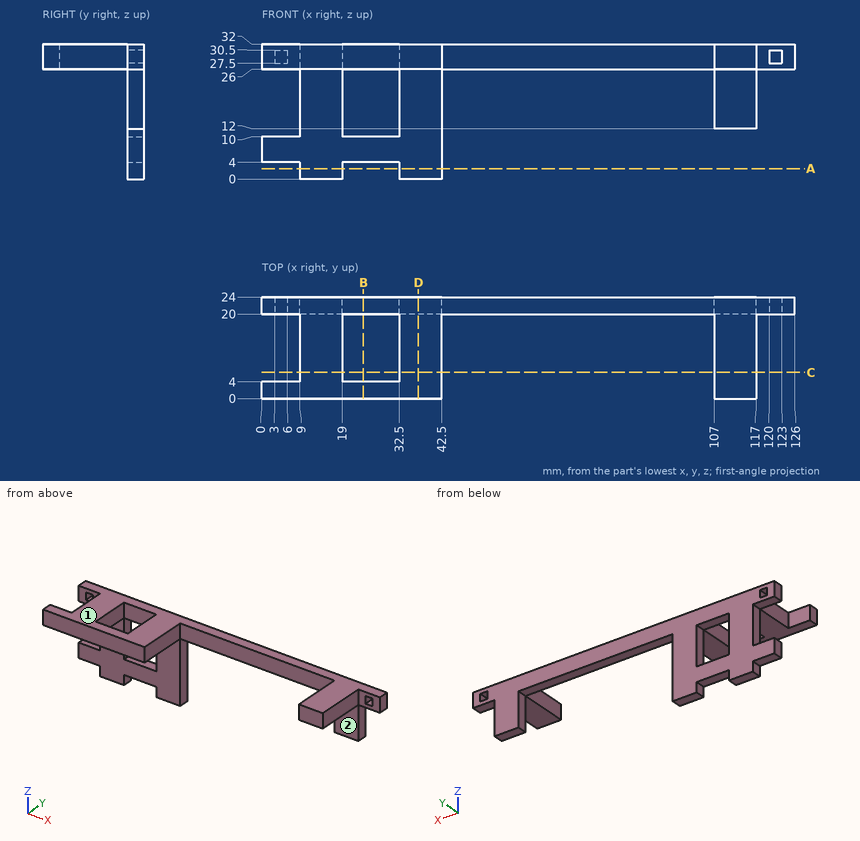
Study the drawing (mm; zero at the part's minimum x, y, z) and answer. A direction names the side the tool comes from. Round coordinates to 2 decimals unless told otherwise and drop trailing zeros. Loops run counter-clockwise (first coordinate to the right, second up) from the corner with the lowest first, then second, coordinate; pieces in that order, holes last.
Q1. Section D-D, the plane x = 37 is taken. Determine the outline of the cut face in (y, z), then the cut area to 3 significant figures.
Q2. Which of the six approach directions +Z, -Z, +X, -X, +Y, -Y give full straight-line access (tool end or side, diameter ignored) to the marked faces 1 and 2?
Q3. Find the intervals of material crossed by line 1 (X direction, y = 20.25, z = 21); line 2 (X direction, y = 3, z = 27.5); line 3 (Z direction, x = 39, y = 15.25), in increasing order.
Q4. Section C-C, the plane y = 6.25 is taken. Determine the outline of the cut face in (x, z), then the cut area to 3 significant figures.
Q5. Section A-A, the plane z = 2.5 is taken. Determine the outline of the cut face in (x, y).
Q6. Section B-B, the plane x = 24 is taken. Determine the outline of the cut face in (y, z).
Q7. Given pin 1 Ø1.8 at (x, z) = (75, 28) entering from -Y; pin 2 Ø1.2 at (x, y) = (25.5, 22) entering from -Z; pin 3 Ø5 at (y, z) = (6.5, 30.5) entering from +X, each flat-ended and moving along its own axis, determine where each tip first touches the part or whether it passes through.
Completed:
1. outline: (0, 26) - (20, 26) - (20, 0) - (24, 0) - (24, 32) - (0, 32) - close
1. area: 248 mm2
2. face 1: +Z, +X, -X, +Y, -Y
2. face 2: -Z, +X, -X, -Y
3. line 1: x = 9 to 19, 32.5 to 42.5, 107 to 117
3. line 2: x = 0 to 42.5, 107 to 117
3. line 3: z = 26 to 32
4. outline: (9, 26) - (19, 26) - (19, 32) - (9, 32) - close; (32.5, 26) - (42.5, 26) - (42.5, 32) - (32.5, 32) - close; (107, 26) - (117, 26) - (117, 32) - (107, 32) - close
4. area: 180 mm2
5. outline: (9, 20) - (19, 20) - (19, 24) - (9, 24) - close; (32.5, 20) - (42.5, 20) - (42.5, 24) - (32.5, 24) - close
6. outline: (0, 26) - (4, 26) - (4, 32) - (0, 32) - close; (20, 4) - (24, 4) - (24, 10) - (20, 10) - close; (20, 26) - (24, 26) - (24, 32) - (20, 32) - close
7. pin 1: stops at y = 20
7. pin 2: stops at z = 4
7. pin 3: stops at x = 117
